Work out the finished part from the listing and answer in its coordinate system (mm). Give positions to 0.01 mm unless a question says otherwise; leave off trailing zeros. Loops run counter-clockwise (first coordinate to the right, second up) from the corner with the lowest first, then second, coordinate; pieces in that order, holes last.
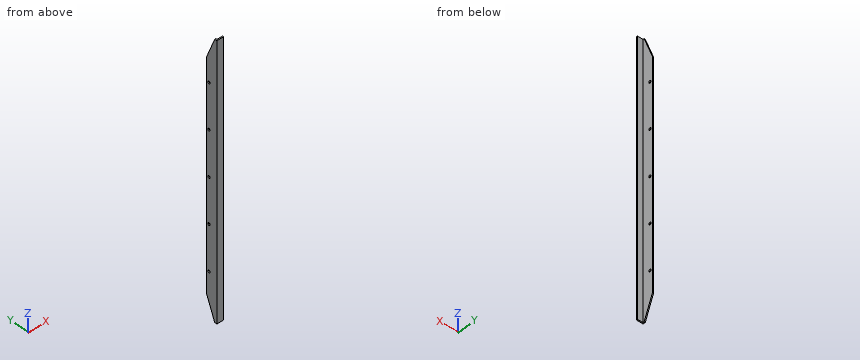
```python
from build123d import *

# Parameters (mm, degrees)
EXTRUDE_THIN1_DEPTH         = 1511.3
F_1_2_CLEARANCE_HOLE1_D     = 13.89126
F_1_2_CLEARANCE_HOLE1_DEPTH = 16.51
F_1_2_CLEARANCE_HOLE1_TIP   = 4.173355541
CUT_EXTRUDE1_DEPTH          = 6.35


with BuildPart() as part:
    # Sketch1 → Extrude-Thin1 (new body)
    with BuildSketch(Plane.XY):
        Polygon((0, 63.5), (0, 0), (38.1, 0), (38.1, 6.35), (6.35, 6.35), (6.35, 63.5), align=None)
    extrude(amount=EXTRUDE_THIN1_DEPTH)

    # 1/2 Clearance Hole1
    with Locations(Plane.ZY):
        with Locations((1259.416666667, 47.625), (1007.533333333, 47.625), (755.65, 47.625), (503.766666667, 47.625), (251.883333333, 47.625)):
            Hole(F_1_2_CLEARANCE_HOLE1_D / 2, depth=F_1_2_CLEARANCE_HOLE1_DEPTH)
            with Locations((0, 0, -(F_1_2_CLEARANCE_HOLE1_DEPTH + F_1_2_CLEARANCE_HOLE1_TIP / 2))):  # 118° drill point
                Cone(0, F_1_2_CLEARANCE_HOLE1_D / 2, F_1_2_CLEARANCE_HOLE1_TIP, mode=Mode.SUBTRACT)

    # Sketch4 → Cut-Extrude1 (cut)
    with BuildSketch(Plane.ZY):
        Polygon((1511.3, 12.7), (1384.3, 63.5), (1511.3, 63.5), align=None)
        Polygon((127, 63.5), (0, 12.7), (0, 63.5), align=None)
    extrude(amount=-CUT_EXTRUDE1_DEPTH, mode=Mode.SUBTRACT)


solid = part.part
```
Q1. Section B-B on x = 15 is taken. Give the vertices of the cut face in (y, z), plus the area to 3 significant figures.
Q2. Consider line 1 along Y through (x, z) = (20.5, 363). Determine where the line is inside the solid, lowest interval first.
Q3. Section A-A on z = 440 is taken. Give the vertices of the cut face in (x, y), plus the area to 3 significant figures.
Q4. Given pin 1 (5 mm diameter, centred on y = 45.5, z = 594.5, fed in from +X), flat-ended and moving along its own axis, determine where the tip first touches the part or whether it passes through.
Check result:
1. outline: (0, 0) - (6.35, 0) - (6.35, 1511.3) - (0, 1511.3) - close
1. area: 9,600 mm2
2. line 1: y = 0 to 6.35
3. outline: (0, 0) - (38.1, 0) - (38.1, 6.35) - (6.35, 6.35) - (6.35, 63.5) - (0, 63.5) - close
3. area: 605 mm2
4. pin 1: stops at x = 6.35
